Check sheet for the drawn part. Datum: minimum x, y, z corner. Units: mm. A direction names the side the tool comes from. Coordinates: 2 decimals unless noted, no trailing zeros. Loops run counter-clockwise (first coordinate to the right, second up) from the corner with the lowest first, then second, coordinate; pieces in that order, holes last.
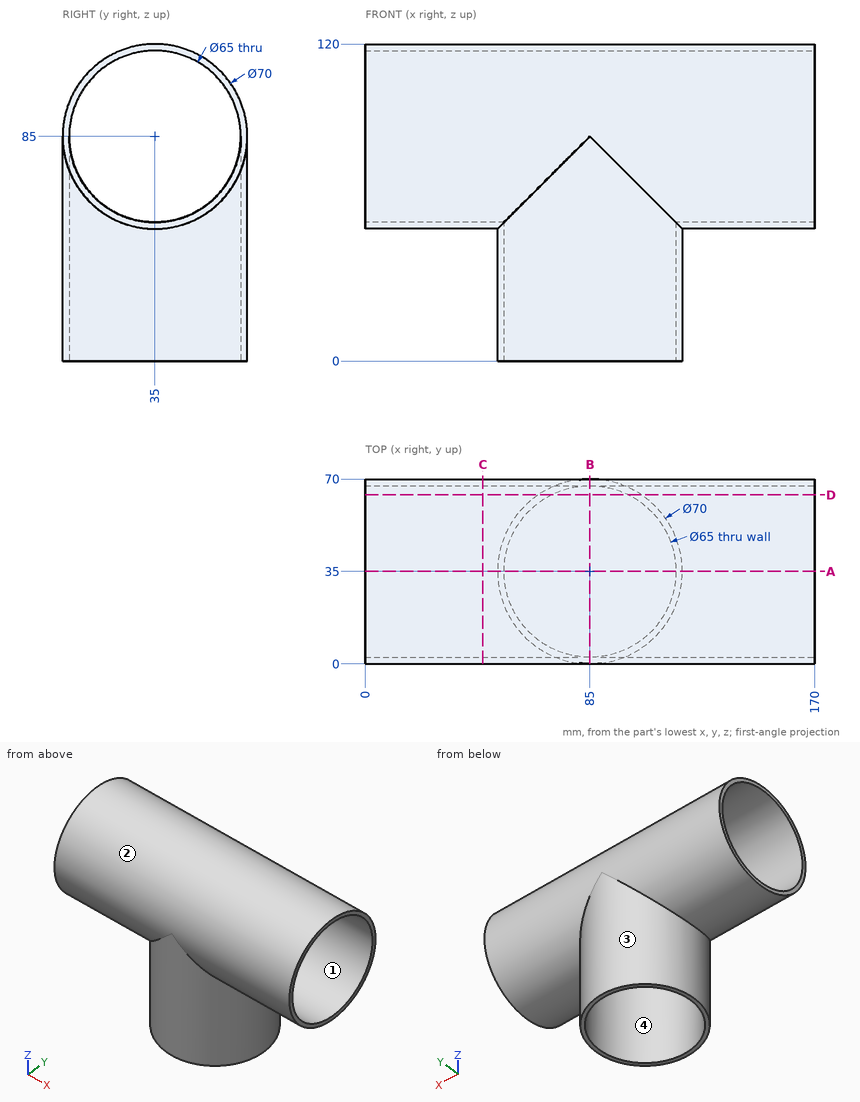
(1) Sectioned sample at B-B on x = 85. Record the cut outline in (y, z).
Findings:
outline: (0, 0) - (2.5, 0) - (2.5, 85) arc R32.5 cw to (67.5, 85) - (67.5, 0) - (70, 0) - (70, 85) arc R35 ccw to (0, 85) - close
(2) Gauge pin test, flat ends, axial feed: pin 1 Ø4 at (x, y) = (60, 18.5) entering from +Z; pin 2 Ø2 at (x, z) = (57, 45) entering from +Y; pin 3 Ø12 at (y, z) = (18.5, 39) entering from -X. Record the tip position at first contact, or that the pin passes through.
Findings:
pin 1: stops at z = 116.86
pin 2: stops at y = 57.27
pin 3: stops at x = 51.61
(3) Scan lines: L1, parallel to Y at x = 83, z = 85; L2, parallel to X at y = 35, z = 24; L3, parallel to Z at x = 14.5, y = 33.5. Record each from-to range of solid material in increasing order.
Findings:
L1: y = 0 to 2.5, 67.5 to 70
L2: x = 50 to 52.5, 117.5 to 120
L3: z = 50.03 to 52.53, 117.47 to 119.97
(4) Sectioned sample at A-A on y = 35. Record the cut outline in (x, z), and give its area (4 significant figures).
Findings:
outline: (0, 50) - (50, 50) - (50, 0) - (52.5, 0) - (52.5, 52.5) - (0, 52.5) - close; (0, 117.5) - (170, 117.5) - (170, 120) - (0, 120) - close; (117.5, 0) - (120, 0) - (120, 50) - (170, 50) - (170, 52.5) - (117.5, 52.5) - close
area: 937.5 mm2
(5) Access from +Z, -Z, +X, -X, +Y, -Y to the whole of each face (thin tool, end or side, straight path). Record for the marked faces 1 and 2.
Findings:
face 1: +X, -X
face 2: none
(6) Draft check along X on the marked faces 3 and 4. Enter one of: +X half, -X half, draft (parallel to the pull), parting line (faces both ways), or undercut.
Findings:
face 3: parting line
face 4: undercut
(7) Sectioned sample at D-D on y = 64. Record the cut outline in (x, z), and give its area (3 significant figures).
Findings:
outline: (0, 65.4) - (65.4, 65.4) - (65.4, 0) - (70.33, 0) - (70.33, 70.33) - (0, 70.33) - close; (0, 99.67) - (170, 99.67) - (170, 104.6) - (0, 104.6) - close; (99.67, 0) - (104.6, 0) - (104.6, 65.4) - (170, 65.4) - (170, 70.33) - (99.67, 70.33) - close
area: 2,170 mm2
(8) Sectioned sample at C-C on x = 44.5. Record the cut outline in (y, z).
Findings:
outline: circle Ø70 at (35, 85); hole circle Ø65 at (35, 85)
